from build123d import *

# Parameters (mm, degrees)
SKETCH1_R           = 15
BOSS_EXTRUDE1_DEPTH = 0.8
CUT_EXTRUDE1_DEPTH  = 1.8


with BuildPart() as part:
    # Sketch1 → Boss-Extrude1 (new body)
    with BuildSketch(Plane(origin=(0, 0, 0), x_dir=(1, 0, 0), z_dir=(0, 1, 0))):
        Circle(SKETCH1_R)
    extrude(amount=BOSS_EXTRUDE1_DEPTH)

    # Sketch3 → Cut-Extrude1 (cut, through all)
    with BuildSketch(Plane(origin=(0, 0.8, 0), x_dir=(1, 0, 0), z_dir=(0, 1, 0))):
        with BuildLine():
            Line((6.32455532, -1.5), (11.5, -1.5))
            ThreePointArc((11.5, -1.5), (13, 0), (11.5, 1.5))
            Line((11.5, 1.5), (6.32455532, 1.5))
            ThreePointArc((6.32455532, 1.5), (-6.5, 0), (6.32455532, -1.5))
        make_face()
    extrude(amount=-CUT_EXTRUDE1_DEPTH, mode=Mode.SUBTRACT)


solid = part.part
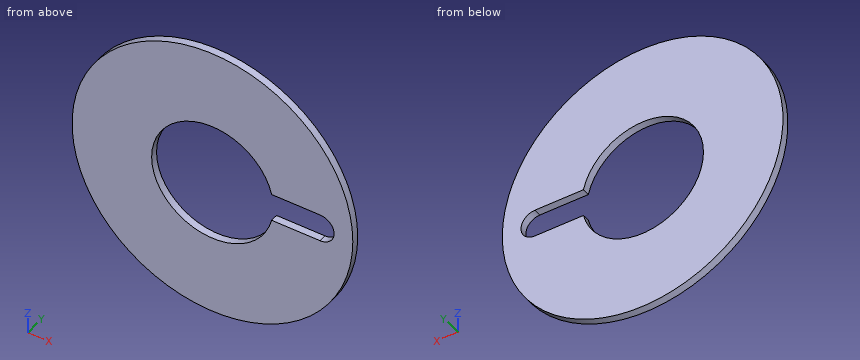
Can you work these out from the model? Positions are in its coordinate system, mm. Coordinates: 2 decimals unless noted, no trailing zeros. Loops run counter-clockwise (first coordinate to the right, second up) from the corner with the lowest first, then second, coordinate; pieces in that order, holes last. Notation, with made-up numbers: (13, 85.5) - (25, 85.5) arc R37 cw to (25, 124.5) - close; hole circle Ø2 at (-30.75, 86). An arc over 180 degrees is marked (long way). Put each result on its own line as item: value. Start each with the question number.
Item 1: Suppose I cut it at A-A (x = 9). Please give me the cut outline in (y, z).
Item 2: If I drill on line 1 along Z through (x, y) = (0, 0.4); line 2 along X through (y, z) = (0.2, 0); line 3 along X through (y, z) = (0.6, -3.5), over which ranges is the centre line in solid material (lowest first)?
Item 3: Suppose I cut it at D-D (z = 7.25). Please give me the cut outline in (x, y).
Item 4: Suppose I cut it at C-C (y = 0.2). Please give me the cut outline in (x, z).
Item 5: Suppose I cut it at B-B (z = 0). Please give me the cut outline in (x, y), and give its area (3 significant figures).
Here are the results:
1. outline: (0, -12) - (0.8, -12) - (0.8, -1.5) - (0, -1.5) - close; (0, 1.5) - (0.8, 1.5) - (0.8, 12) - (0, 12) - close
2. line 1: -15 to -6.5, 6.5 to 15
2. line 2: -15 to -6.5, 13 to 15
2. line 3: -14.59 to -5.48, 5.48 to 14.59
3. outline: (-13.13, 0) - (13.13, 0) - (13.13, 0.8) - (-13.13, 0.8) - close
4. outline: circle Ø30 at (0, 0); hole (6.32, -1.5) - (11.5, -1.5) arc R1.5 ccw to (11.5, 1.5) - (6.32, 1.5) arc R6.5 ccw (long way) to start
5. outline: (-15, 0) - (-6.5, 0) - (-6.5, 0.8) - (-15, 0.8) - close; (13, 0) - (15, 0) - (15, 0.8) - (13, 0.8) - close
5. area: 8.40 mm²
